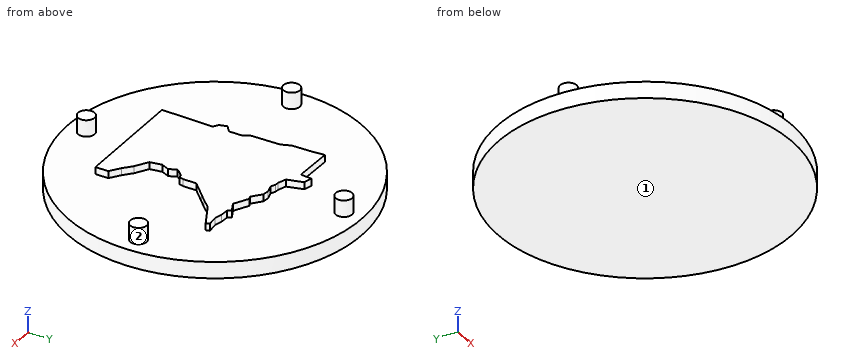
```python
from build123d import *

# Parameters (mm, degrees)
F0_R     = 15.875
F1_DEPTH = 1.778
F3_R     = 0.889
F4_DEPTH = 1.778
F6_DEPTH = 0.762


with BuildPart() as f1:
    # F0 (on Top) → F1 (new body)
    with BuildSketch(Plane.XY):
        Circle(F0_R)
    extrude(amount=-F1_DEPTH)

    # F3 (on face) → F4 (join)
    with BuildSketch(Plane.XY):
        with Locations((0, 13.836063)):
            Circle(F3_R)
        with Locations((-13.862842, 0)):
            Circle(F3_R)
        with Locations((-0.025139, -13.808045)):
            Circle(F3_R)
        with Locations((13.819266, 0)):
            Circle(F3_R)
    extrude(amount=F4_DEPTH)

    # F5 (on face) → F6 (join)
    with BuildSketch(Plane.XY):
        Polygon((-2.453811, 8.900641), (-2.5601, 7.696021), (-6.669981, 7.837741), (-6.563691, 6.455971), (-6.528262, 4.365601), (-6.138531, 3.338131), (-6.103101, 0.114), (-5.713371, -0.55917), (-5.713371, -1.87008), (-6.421971, -2.47239), (-6.209391, -3.251851), (-5.677941, -3.606151), (-5.819661, -9.133232), (5.978531, -9.274952), (5.978531, -7.893181), (4.915631, -7.113722), (4.029881, -6.298832), (2.68354, -5.448511), (2.47096, -4.173031), (2.860691, -3.322711), (2.47096, -2.54325), (2.82526, -2.11809), (3.17956, -1.76379), (3.53386, -1.69293), (3.675581, -1.23234), (3.675581, 0.18486), (5.128211, 1.60206), (5.872241, 2.31066), (6.687131, 3.196411), (9.273522, 4.507321), (9.167232, 4.897051), (8.068902, 4.790761), (7.254011, 5.003341), (6.368261, 5.074201), (6.084821, 5.428501), (5.057351, 4.932481), (3.53386, 5.782801), (3.17956, 5.641081), (2.18752, 6.491401), (1.51435, 6.597691), (0.66403, 6.349681), (0.16801, 6.597691), (-0.25715, 6.633121), (-1.10747, 6.951991), (-1.56806, 8.652632), align=None)
    extrude(amount=F6_DEPTH)


solid = f1.part
```
For this review, take the finished solid that the model builds, in its own axes (mm). Face numbers are marked on the shaded views. A direction names the side the tool comes from. Coordinates: 2 decimals unless noted, no trailing zeros. Loops run counter-clockwise (first coordinate to the right, second up) from the corner with the lowest first, then second, coordinate; pieces in that order, holes last. Notation, with made-up numbers: (77, 45.5) -> (103, 45.5) arc R37 ccw to (103, 81.5) -> close; hole circle Ø7 at (16.25, 77.5). An arc over 180 degrees is marked (long way). Return JSON: item names as keys, results as strings. Group by question number.
(1) Consider section B-B, the plane y = 12.5. Give the boundary of the cut face in (x, z), plus the area to 3 significant figures.
(2) Consider section A-A, the plane z = -0.85. Give the boundary of the cut face in (x, y) (3 decimals).
(3) For pin 1 Ø12 at (x, y) = (-0.5, -0.5) entering from +Z; pin 2 Ø4 at (x, y) = (-8.5, -2) entering from +Z; pin 3 Ø0.6 at (y, z) = (-1, 0) entering from -X, all flat-tipped, find the tip position at first contact; note any pin that passes through.
(4) To check wall thickness, follow L1, parallel to Z at x = 3, y = -1; L2, parallel to Z at x = -15, y = 2; L3, parallel to X at y = 14.5, z = -1.2. State the ranges of each line that lie inside material, in increasing order.
(5) Tool access review of the marked faces 1 and 2: name each direction out of +Z, -Z, +X, -X, +Y, -Y from which nothing blocks a thin tool from reaching the whole face with its end or side.
(6) Consider section C-C, the plane y = -11. Give the boundary of the cut face in (x, z), plus the area to 3 significant figures.
Results below:
{
 "1": {"outline": "(-9.79, -1.78) -> (9.79, -1.78) -> (9.79, 0) -> (-9.79, 0) -> close", "area": "34.8 mm2"},
 "2": {"outline": "circle Ø31.75 at (0, 0)"},
 "3": {"pin 1": "stops at z = 0.76", "pin 2": "stops at z = 0", "pin 3": "stops at x = -15.86"},
 "4": {"L1": "z = -1.78 to 0.76", "L2": "z = -1.78 to 0", "L3": "x = -6.46 to 6.46"},
 "5": {"face 1": "-Z, +X, -X, +Y, -Y", "face 2": "+Z"},
 "6": {"outline": "(-11.45, -1.78) -> (11.45, -1.78) -> (11.45, 0) -> (-11.45, 0) -> close", "area": "40.7 mm2"}
}
